The listing builds one solid part. Answer for the finished solid, in the listing's coordinates (mm). A direction names the side the tool comes from. Coordinates: 2 decimals unless noted, no trailing zeros. Order: outer loops, then holes, each group sorted by start corner. A loop starts at its lowest first (then second) coordinate and runs counter-clockwise, first axis right, second up. Notation, with made-up numbers: (42, 35.25) -> (80, 35.25) arc R25 ccw to (80, 56.25) -> close; hole circle Ø7 at (4.25, -35.5). An arc over 180 degrees is marked (long way). Return JSON: item names as keys, results as strings.
from build123d import *
from OCP.BRepFilletAPI import BRepFilletAPI_MakeChamfer

# Parameters (mm, degrees)
EXTRUDE_1_DEPTH     = 26
SKETCH_2_R          = 1.65
CUT_EXTRUDE_1_DEPTH = 45.819078563
SKETCH_3_W          = 28.1444964
SKETCH_3_H          = 6.1
CUT_EXTRUDE_2_DEPTH = 35.940261345
CUT_EXTRUDE_4_REACH = 46.819
SKETCH_5_R          = 4.1
SKETCH_6_R          = 1.65
CUT_EXTRUDE_5_DEPTH = 41.050210522
CHAMFER_1_SIZE      = 2
CHAMFER_1_SIZE2     = 11.342563639
FILLET_1_R          = 2


with BuildPart() as part:
    # 草图1 → 凸台-拉伸1 (new body)
    with BuildSketch(Plane(origin=(0, 0, 0), x_dir=(0, 0, -1), z_dir=(1, 0, 0))):
        with BuildLine():
            Line((17.407451211, 15.55), (2.245544981, 15.55))
            Line((2.245544981, 15.55), (-2.273793452, 10))
            Line((-2.273793452, 10), (-10.273793452, 10))
            Line((-10.273793452, 10), (-13.270509165, 6.44212097))
            ThreePointArc((-13.270509165, 6.44212097), (-15.622040206, 0), (-13.270509165, -6.44212097))
            Line((-13.270509165, -6.44212097), (-10.273793452, -10))
            Line((-10.273793452, -10), (-2.273793452, -10))
            Line((-2.273793452, -10), (2.245544981, -15.55))
            Line((2.245544981, -15.55), (17.407451211, -15.55))
            Line((17.407451211, -15.55), (17.407451211, 15.55))
        make_face()
        with BuildLine():
            Line((3.687588487, 12.45), (14.307451211, 12.45))
            Line((14.307451211, 12.45), (14.307451211, -12.45))
            Line((14.307451211, -12.45), (3.687588487, -12.45))
            Line((3.687588487, -12.45), (-3.977203858, -3.349902904))
            ThreePointArc((-3.977203858, -3.349902904), (-5.2, 0), (-3.977203858, 3.349902904))
            Line((-3.977203858, 3.349902904), (3.687588487, 12.45))
        make_face(mode=Mode.SUBTRACT)
    extrude(amount=EXTRUDE_1_DEPTH)

    # 草图2 → 切除-拉伸1 (cut, through all)
    with BuildSketch(Plane(origin=(0, 0, -17.407451211), x_dir=(-1, 0, 0), z_dir=(0, 0, -1))):
        with Locations((-22.5, 5.5)):
            Circle(SKETCH_2_R)
        with Locations(Location((-22.5, -5.5, 0), (0, 0, 325.181239638))):
            Circle(SKETCH_2_R)
        with Locations(Location((-3.5, -5.5, 0), (0, 0, 325.181239638))):
            Circle(SKETCH_2_R)
        with Locations(Location((-3.5, 5.5, 0), (0, 0, 180))):
            Circle(SKETCH_2_R)
    extrude(amount=-CUT_EXTRUDE_1_DEPTH, mode=Mode.SUBTRACT)

    # 草图3 → 切除-拉伸2 (cut, through all)
    with BuildSketch(Plane.ZY):
        with Locations((-3.335203011, -12.5)):
            Rectangle(SKETCH_3_W, SKETCH_3_H)
    extrude(amount=-CUT_EXTRUDE_2_DEPTH, mode=Mode.SUBTRACT)

    # 草图5 → 切除-拉伸4 (cut, up to next)
    with BuildSketch(Plane.XY.offset(15.622040206), mode=Mode.PRIVATE) as cut_extrude_4_sk1:
        with Locations(Location((13, -3.65, 0), (0, 0, 4.197484636))):
            Circle(SKETCH_5_R)
    cut_extrude_4_tool1 = extrude(cut_extrude_4_sk1.sketch, amount=-CUT_EXTRUDE_4_REACH, mode=Mode.PRIVATE) & part.part
    add(cut_extrude_4_tool1.solids().sort_by_distance((13, -3.65, 15.62204))[0], mode=Mode.SUBTRACT)

    # 草图6 → 切除-拉伸5 (cut, through all)
    with BuildSketch(Plane.XZ.offset(9.45)):
        with Locations(Location((13, 4.737045189, 0), (0, 0, 270))):
            Circle(SKETCH_6_R)
    extrude(amount=-CUT_EXTRUDE_5_DEPTH, mode=Mode.SUBTRACT)

    # 倒角1: one chamfer whose edges measure the first distance from different faces: ONE call of the kernel's chamfer builder (chamfer() names one face for all edges)
    chamfer_1_edges_1 = [part.edges().sort_by_distance(p)[0] for p in [
        (0, -9.45, 4.78814218),
    ]]
    chamfer_1_side_1 = [part.faces().sort_by_distance(p)[0] for p in [
        (0, -9.035760057, -15.857451211),
    ]]
    chamfer_1_edges_2 = [part.edges().sort_by_distance(p)[0] for p in [
        (26, -9.45, 4.78814218),
    ]]
    chamfer_1_side_2 = [part.faces().sort_by_distance(p)[0] for p in [
        (26, -9.035760057, -15.857451211),
    ]]
    chamfer_1 = BRepFilletAPI_MakeChamfer(part.part.solid().wrapped)
    for e in chamfer_1_edges_1:
        chamfer_1.Add(CHAMFER_1_SIZE, CHAMFER_1_SIZE2, e.wrapped, chamfer_1_side_1[0].wrapped)  # the first distance lies on this face
    for e in chamfer_1_edges_2:
        chamfer_1.Add(CHAMFER_1_SIZE, CHAMFER_1_SIZE2, e.wrapped, chamfer_1_side_2[0].wrapped)  # the first distance lies on this face
    add(Compound.cast(chamfer_1.Shape()), mode=Mode.REPLACE)

    # 圆角1
    # the kernel refuses this fillet: 2 mm, written as the material it takes off along each edge
    with BuildSketch(Plane(origin=(26, -7.45, -3.671707212), x_dir=(-0.9848077530122086, -0.17364817766692747, 0), z_dir=(0, 0, 1))) as fillet_1_piece_1:
        with BuildLine():
            CenterArc((FILLET_1_R * 0.839099631177, -FILLET_1_R), FILLET_1_R, 90, 80)
            Line((-FILLET_1_R * 0.145708121835, -FILLET_1_R * 0.826351822333), (0, 0))
            Line((0, 0), (FILLET_1_R * 0.839099631177, 0))
        make_face()
    extrude(amount=20.288802329, mode=Mode.SUBTRACT)
    with BuildSketch(Plane(origin=(0, -7.45, 16.617095117), x_dir=(0, 1, 0), z_dir=(0, 0, -1))) as fillet_1_piece_2:
        with BuildLine():
            CenterArc((FILLET_1_R * 0.839099631177, FILLET_1_R), FILLET_1_R, 190, 80)
            Line((-FILLET_1_R * 0.145708121835, FILLET_1_R * 0.826351822333), (0, 0))
            Line((0, 0), (FILLET_1_R * 0.839099631177, 0))
        make_face()
    extrude(amount=20.288802329, mode=Mode.SUBTRACT)


solid = part.part
1. Each of these flat-tipped pins is pushed along its axis until it touches: pin 1 Ø2.5 at (x, y) = (3.5, 5.5) entering from +Z; pin 2 Ø8 at (x, y) = (8, 12) entering from +Z; pin 3 Ø4.5 at (x, y) = (3.5, -5.5) entering from +Z; pin 4 Ø4 at (x, z) = (9, 8) entering from +Y. Where does it stop, or does it pass through?
Answer block:
{"pin 1": "passes through", "pin 2": "stops at z = 11.96", "pin 3": "stops at z = 15.08", "pin 4": "stops at y = 10"}
2. Determine the mould class of faces 6 (the face through (13, 3, -17.407)), 7 (the face through (13, 2, -14.307)), 8 (the face through (21.61, 6.89, 7.7)) for opening direction Z: pulls with the +Z half, pulls with the -Z half, needs draft (parallel to the pull), parting line crosses it, or undercut.
Answer block:
{"face 6": "pulls with the -Z half", "face 7": "undercut", "face 8": "needs draft"}
3. The part is cut by section C-C on y = 2. Give the vertices of the cut face in (x, z).
Answer block:
{"outline": "(0, -17.41) -> (26, -17.41) -> (26, -14.31) -> (0, -14.31) -> close; (0, 4.8) -> (11.35, 4.8) arc R1.65 cw to (14.65, 4.8) -> (26, 4.8) -> (26, 15.42) -> (0, 15.42) -> close"}
4. The part is cut by section D-D on z = 3.5. Give the number of separate pieces and of enclosed holes in the cut face, and give its area (3 significant figures).
Answer block:
{"separate pieces": "4", "enclosed holes": "0", "area": "203 mm2"}
5. The part is cut by section B-B on x = 13. Give the vertices of the cut face in (y, z), and give its area (3 significant figures).
Answer block:
{"outline": "(-9.45, -17.41) -> (15.55, -17.41) -> (15.55, -2.25) -> (10, 2.27) -> (10, 3.09) -> (4.41, 3.09) -> (12.45, -3.69) -> (12.45, -14.31) -> (-9.45, -14.31) -> close; (-9.45, -1.16) -> (-7.75, 0.27) -> (-7.75, 3.09) -> (-9.45, 3.09) -> close; (-9.45, 6.39) -> (-7.75, 6.39) -> (-7.75, 12.17) -> (-9.45, 10.74) -> close; (0.45, 6.39) -> (10, 6.39) -> (10, 10.27) -> (6.44, 13.27) arc R10 ccw to (0.45, 15.61) -> close", "area": "226 mm2"}
6. Consider line 1 (Y direction, x = 3.5, z = -16.15); line 2 (X direction, y = -5.5, z = -16.5); line 3 (X direction, y = -3.65, z = 10.75). Determine where each line is inside the solid, lowest interval first. Write a range as from..to.
Answer block:
{"line 1": "y = -9.45..-7.15, -3.85..3.85, 7.15..15.55", "line 2": "x = 0..1.85, 5.15..20.85, 24.15..26", "line 3": "x = 0..8.9, 17.1..26"}
7. The part is cut by section A-A on y = 5.5. Give the vertices of the cut face in (x, z).
Answer block:
{"outline": "(0, -17.41) -> (1.85, -17.41) -> (1.85, -14.31) -> (0, -14.31) -> close; (0, 2.17) -> (1.85, 2.17) -> (1.85, 13.97) -> (0, 13.97) -> close; (5.15, -17.41) -> (20.85, -17.41) -> (20.85, -14.31) -> (5.15, -14.31) -> close; (5.15, 2.17) -> (20.85, 2.17) -> (20.85, 13.97) -> (5.15, 13.97) -> close; (24.15, -17.41) -> (26, -17.41) -> (26, -14.31) -> (24.15, -14.31) -> close; (24.15, 2.17) -> (26, 2.17) -> (26, 13.97) -> (24.15, 13.97) -> close; hole circle Ø3.3 at (13, 4.74)"}
8. For faces 1 (the face through (13, -9.45, -16)), 2 (the face through (5.7, -0.1, 5.2)), 3 (the face through (12.818, 1.646, 15.486)), 4 (the face through (0.48, -7.07, 7.13)), 5 (the face through (13, 12.45, -9)), determine the directions among +Z, -Z, +X, -X, +Y, -Y from which every point of the face is accessible in a straight line to the end or side of a thin tool.
Answer block:
{"face 1": "+Z, -Z, +X, -X, -Y", "face 2": "+X, -X", "face 3": "+Z, +X, -X", "face 4": "+Z, -X, -Y", "face 5": "+X, -X, -Y"}
